```python
from build123d import *

# Parameters (mm, degrees)
SKETCH1_R           = 2.45745
BOSS_EXTRUDE1_DEPTH = 9.525


with BuildPart() as part:
    # Sketch1 → Boss-Extrude1 (new body)
    with BuildSketch(Plane(origin=(0, 0, 0), x_dir=(1, 0, 0), z_dir=(0, 1, 0))):
        with BuildLine():
            Line((0, 0), (965.2, 0))
            Line((965.2, 0), (965.2, 69.85))
            Line((965.2, 69.85), (952.5, 69.85))
            Line((952.5, 69.85), (952.5, 63.5))
            ThreePointArc((952.5, 63.5), (945.060512242, 45.539487758), (927.1, 38.1))
            Line((927.1, 38.1), (669.925, 38.1))
            ThreePointArc((669.925, 38.1), (651.964487758, 45.539487758), (644.525, 63.5))
            Line((644.525, 63.5), (644.525, 69.85))
            Line((644.525, 69.85), (636.5875, 69.85))
            Line((636.5875, 69.85), (636.5875, 63.5))
            ThreePointArc((636.5875, 63.5), (629.148012242, 45.539487758), (611.1875, 38.1))
            Line((611.1875, 38.1), (354.0125, 38.1))
            ThreePointArc((354.0125, 38.1), (336.051987758, 45.539487758), (328.6125, 63.5))
            Line((328.6125, 63.5), (328.6125, 69.85))
            Line((328.6125, 69.85), (320.675, 69.85))
            Line((320.675, 69.85), (320.675, 63.5))
            ThreePointArc((320.675, 63.5), (313.235512242, 45.539487758), (295.275, 38.1))
            Line((295.275, 38.1), (38.1, 38.1))
            ThreePointArc((38.1, 38.1), (20.139487758, 45.539487758), (12.7, 63.5))
            Line((12.7, 63.5), (12.7, 69.85))
            Line((12.7, 69.85), (0, 69.85))
            Line((0, 69.85), (0, 0))
        make_face()
        with Locations((69.85, 15.875)):
            Circle(SKETCH1_R, mode=Mode.SUBTRACT)
        with Locations((345.01582, 15.875)):
            Circle(SKETCH1_R, mode=Mode.SUBTRACT)
        with Locations((895.35, 15.875)):
            Circle(SKETCH1_R, mode=Mode.SUBTRACT)
        with Locations((620.18418, 15.875)):
            Circle(SKETCH1_R, mode=Mode.SUBTRACT)
    extrude(amount=BOSS_EXTRUDE1_DEPTH)


solid = part.part
```
The listing builds one solid part. Answer for the finished solid, in the listing's coordinates (mm). A direction names the side the tool comes from. Round coordinates to 2 decimals unless told otherwise and drop trailing zeros. Order: outer loops, then holes, each group sorted by start corner. A loop starts at its lowest first (then second) coordinate and runs counter-clockwise, first axis right, second up. Notation, with made-up numbers: (-8.5, 77) -> (3.5, 77) arc R30 ccw to (3.5, 103) -> close; hole circle Ø4 at (31, 0.25). An arc over 180 degrees is marked (long way). Answer as CSV lines item,"result". Start each with the question number.
(1) The part is cut by section B-B (x = 391). Determine the outline of the cut face in (y, z) (3 decimals), then the cut area to 3 significant figures.
(2) A tool of negligible diameter and unlimited length cuts with its end or side. For faces 3 (the face through (476, 0, -20)), 4 (the face through (945.26, 4.7, -45.74)), from which of +Z, -Z, +X, -X, +Y, -Y can it reach the whole face along a straight path? Write none if from no direction.
(3) Find the intervals of material crossed by probe 1 along X at (y, z) = (5.5, -58); probe 2 along X at (y, z) = (1.25, -15); probe 3 along X at (y, z) = (1.25, -65) (1 decimal), in increasing order. Write a range as from..to.
(4) Flat-ended cylindrical pins translate along their axes: pin 1 Ø3 at (x, z) = (895.35, -15.875) entering from +Y; pin 2 Ø3 at (x, y) = (123.5, 6.5) entering from -Z. Find the tip coordinate at first contact, or state that the pin passes through.
(5) For a pull along X with two mould halves and no side action, classify faces 1 (the face through (313.432, 4.696, -45.738)), 2 (the face through (476, 9.525, -20)) as +X half, -X half, draft (parallel to the pull), parting line (faces both ways), or undercut.
(6) The part is cut by section A-A (y = 7). Count the separate pieces of the cut face and the enclosed holes in it, then the cut area to 3 significant figures.
Evaluation:
1,outline,"(0, -38.1) -> (9.525, -38.1) -> (9.525, 0) -> (0, 0) -> close"
1,area,"363 mm²"
2,face 3,"+Z, -Z, +X, -X, -Y"
2,face 4,"-Z, +Y, -Y"
3,probe 1,"0..13.3, 320.07..329.22, 635.98..645.13, 951.9..965.2"
3,probe 2,"0..67.55, 72.15..342.72, 347.31..617.89, 622.48..893.05, 897.65..965.2"
3,probe 3,"0..12.7, 320.7..328.6, 636.6..644.5, 952.5..965.2"
4,pin 1,"through"
4,pin 2,"z = -38.1"
5,face 1,"undercut"
5,face 2,"draft"
6,separate pieces,"1"
6,enclosed holes,"4"
6,area,"38,800 mm²"
